Geometry: final body of the model. Coordinates: model frame, mm. Face numbers are marked on the shaded views. Give positions to 0.01 mm unless a question says otherwise; leave off trailing zeros.
Q1. Pin query (flat end, axial travel): pin 1 Ø1.5 at (y, z) = (2, 41.5) entering from -X; pin 2 Ø10 at (x, y) = (110, 6) entering from +Z; pin 3 Ø2.5 at (x, z) = (152.5, 72.5) entering from -Y. Return the tip coordinate at first contact, or that it passes through.
Q2. Mould query, pull axis X, two halves, no side actions, for the marked faces 1 and 2. Classes: +X half, -X half, draft (parallel to the pull), parting line (faces both ways), or undercut.
Q3. Line query: line 1 (Z direction, x = 1, y = 4.5); line 2 (Z direction, x = 152, y = 5.75); line 3 (X direction, y = 9.5, z = -20). Output: solid intervals per line, ascending.
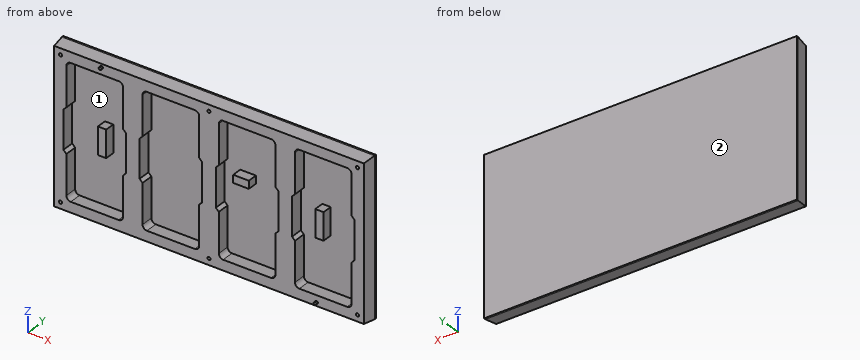
from build123d import *

# Parameters (mm, degrees)
SKETCH2_W                                  = 320
SKETCH2_H                                  = 160
BOSS_EXTRUDE1_DEPTH                        = 2
SKETCH3_R                                  = 1.6
CUT_EXTRUDE1_DEPTH                         = 7
CUT_EXTRUDE2_DEPTH                         = 12.5
MIRROR1_AT_THE_SECOND_PLANE_COPY_1_SKETC_R = 1.6
MIRROR1_AT_THE_SECOND_PLANE_COPY_1_DEPTH   = 7
MIRROR1_AT_THE_SECOND_PLANE_COPY_2_DEPTH   = 12.5
SKETCH4_W                                  = 8.5
SKETCH4_H                                  = 28
SKETCH4_W_2                                = 16
SKETCH4_H_2                                = 8
BOSS_EXTRUDE3_DEPTH                        = 10
SKETCH5_R                                  = 1.5
BOSS_EXTRUDE4_DEPTH                        = 2


with BuildPart() as part:
    # Sketch2 → Boss-Extrude1 (new body)
    with BuildSketch(Plane(origin=(0, 13, 0), x_dir=(1, 0, 0), z_dir=(0, 1, 0))):
        Rectangle(SKETCH2_W, SKETCH2_H)
    extrude(amount=BOSS_EXTRUDE1_DEPTH)

    # Sketch1 → Loft1 section 0
    with BuildSketch(Plane(origin=(0, 0, 0), x_dir=(1, 0, 0), z_dir=(0, 1, 0))):
        with BuildLine():
            Line((-158.5, -78.5), (158.5, -78.5))
            Line((158.5, -78.5), (158.5, 78.5))
            Line((158.5, 78.5), (-158.5, 78.5))
            Line((-158.5, 78.5), (-158.5, -78.5))
        make_face()
    # Sketch2_2 → Loft1 section 1
    with BuildSketch(Plane(origin=(0, 13, 0), x_dir=(1, 0, 0), z_dir=(0, 1, 0))):
        with BuildLine():
            Line((160, -80), (-160, -80))
            Line((-160, -80), (-160, 80))
            Line((-160, 80), (160, 80))
            Line((160, 80), (160, -80))
        make_face()
    loft()

    # Sketch3 → Cut-Extrude1 (cut)
    with BuildSketch(Plane.XZ):
        with Locations(Location((0, 72, 0), (0, 0, 270))):
            Circle(SKETCH3_R)
        with Locations(Location((-152, 72, 0), (0, 0, 270))):
            Circle(SKETCH3_R)
    cut_extrude1 = extrude(amount=-CUT_EXTRUDE1_DEPTH, mode=Mode.SUBTRACT)

    # Sketch3_4 → Cut-Extrude2 (cut)
    with BuildSketch(Plane.XZ):
        with BuildLine():
            Line((-149, 0), (-117, 0))
            Line((-117, 0), (-117, 67.9))
            Line((-117, 67.9), (-141.5, 67.9))
            ThreePointArc((-141.5, 67.9), (-144.681980515, 66.581980515), (-146, 63.4))
            Line((-146, 63.4), (-146, 22.75))
            Line((-146, 22.75), (-149, 19.75))
            Line((-149, 19.75), (-149, 0))
        make_face()
        with BuildLine():
            Line((-117, 0), (-85, 0))
            Line((-85, 0), (-85, 19.75))
            Line((-85, 19.75), (-88, 22.75))
            Line((-88, 22.75), (-88, 63.4))
            ThreePointArc((-88, 63.4), (-89.318019485, 66.581980515), (-92.5, 67.9))
            Line((-92.5, 67.9), (-117, 67.9))
            Line((-117, 67.9), (-117, 0))
        make_face()
        with BuildLine():
            Line((-71, 0), (-7, 0))
            Line((-7, 0), (-7, 19.75))
            Line((-7, 19.75), (-10, 22.75))
            Line((-10, 22.75), (-10, 63.4))
            ThreePointArc((-10, 63.4), (-11.318019485, 66.581980515), (-14.5, 67.9))
            Line((-14.5, 67.9), (-63.5, 67.9))
            ThreePointArc((-63.5, 67.9), (-66.681980515, 66.581980515), (-68, 63.4))
            Line((-68, 63.4), (-68, 22.75))
            Line((-68, 22.75), (-71, 19.75))
            Line((-71, 19.75), (-71, 0))
        make_face()
    cut_extrude2 = extrude(amount=-CUT_EXTRUDE2_DEPTH, mode=Mode.SUBTRACT)

    # Mirror1: Cut-Extrude1, Cut-Extrude2 across plane
    add(cut_extrude1.mirror(Plane.XY), mode=Mode.SUBTRACT)
    add(cut_extrude2.mirror(Plane.XY), mode=Mode.SUBTRACT)

    # Mirror1 at the second plane: Cut-Extrude1, Cut-Extrude2 across plane
    add(cut_extrude1.mirror(Plane(origin=(0, 0, 0), x_dir=(0, 0, 1), z_dir=(1, 0, 0))), mode=Mode.SUBTRACT)
    add(cut_extrude2.mirror(Plane(origin=(0, 0, 0), x_dir=(0, 0, 1), z_dir=(1, 0, 0))), mode=Mode.SUBTRACT)

    # Mirror1 at the second plane copy 1 sketc → Mirror1 at the second plane copy 1 (cut)
    with BuildSketch(Plane(origin=(0, 0, 0), x_dir=(-1, 0, 0), z_dir=(0, -1, 0))):
        with Locations(Location((0, 72, 0), (0, 0, 270))):
            Circle(MIRROR1_AT_THE_SECOND_PLANE_COPY_1_SKETC_R)
        with Locations(Location((-152, 72, 0), (0, 0, 270))):
            Circle(MIRROR1_AT_THE_SECOND_PLANE_COPY_1_SKETC_R)
    extrude(amount=-MIRROR1_AT_THE_SECOND_PLANE_COPY_1_DEPTH, mode=Mode.SUBTRACT)

    # Mirror1 at the second plane copy 2 sketc → Mirror1 at the second plane copy 2 (cut)
    with BuildSketch(Plane(origin=(0, 0, 0), x_dir=(-1, 0, 0), z_dir=(0, -1, 0))):
        with BuildLine():
            Line((-149, 0), (-117, 0))
            Line((-117, 0), (-117, 67.9))
            Line((-117, 67.9), (-141.5, 67.9))
            ThreePointArc((-141.5, 67.9), (-144.681980515, 66.581980515), (-146, 63.4))
            Line((-146, 63.4), (-146, 22.75))
            Line((-146, 22.75), (-149, 19.75))
            Line((-149, 19.75), (-149, 0))
        make_face()
        with BuildLine():
            Line((-117, 0), (-85, 0))
            Line((-85, 0), (-85, 19.75))
            Line((-85, 19.75), (-88, 22.75))
            Line((-88, 22.75), (-88, 63.4))
            ThreePointArc((-88, 63.4), (-89.318019485, 66.581980515), (-92.5, 67.9))
            Line((-92.5, 67.9), (-117, 67.9))
            Line((-117, 67.9), (-117, 0))
        make_face()
        with BuildLine():
            Line((-71, 0), (-7, 0))
            Line((-7, 0), (-7, 19.75))
            Line((-7, 19.75), (-10, 22.75))
            Line((-10, 22.75), (-10, 63.4))
            ThreePointArc((-10, 63.4), (-11.318019485, 66.581980515), (-14.5, 67.9))
            Line((-14.5, 67.9), (-63.5, 67.9))
            ThreePointArc((-63.5, 67.9), (-66.681980515, 66.581980515), (-68, 63.4))
            Line((-68, 63.4), (-68, 22.75))
            Line((-68, 22.75), (-71, 19.75))
            Line((-71, 19.75), (-71, 0))
        make_face()
    extrude(amount=-MIRROR1_AT_THE_SECOND_PLANE_COPY_2_DEPTH, mode=Mode.SUBTRACT)

    # Sketch4 → Boss-Extrude3 (add)
    with BuildSketch(Plane.XZ.offset(-12.5)):
        with Locations((-111.25, 0)):
            Rectangle(SKETCH4_W, SKETCH4_H)
        with Locations((31, 13)):
            Rectangle(SKETCH4_W_2, SKETCH4_H_2)
        with Locations((111.25, 0)):
            Rectangle(SKETCH4_W, SKETCH4_H)
    extrude(amount=BOSS_EXTRUDE3_DEPTH)

    # Sketch5 → Boss-Extrude4 (add)
    with BuildSketch(Plane.XZ):
        with Locations(Location((-110, 75, 0), (0, 0, 270))):
            Circle(SKETCH5_R)
        with Locations(Location((110, -75, 0), (0, 0, 270))):
            Circle(SKETCH5_R)
    extrude(amount=BOSS_EXTRUDE4_DEPTH)


solid = part.part
Computed:
1. pin 1: stops at x = -158.82
1. pin 2: stops at z = 79.77
1. pin 3: stops at y = 0
2. face 1: undercut
2. face 2: draft
3. line 1: z = -79.02 to -73.25, -70.75 to 70.75, 73.25 to 79.02
3. line 2: z = -79.16 to -73.6, -70.4 to 70.4, 73.6 to 79.16
3. line 3: x = -159.6 to -148.75, -85.25 to -70.75, -7.25 to 7.25, 70.75 to 85.25, 148.75 to 159.6
